Check sheet for the drawn part. Datum: minimum x, y, z corner. Units: mm. A direction names the side the tool comes from. Give positions to 0.01 mm unless a question says otherwise; leave off trailing zeros. Write each loop counter-clockwise with the first axis right and the second up, starting at its lowest first coordinate (ties: lowest second). Pieces come first, ordered by that corner, then holes. Notation, with made-up numbers: (37.25, 72.25) -> (78.25, 72.25) arc R15 cw to (78.25, 79.25) -> close; hole circle Ø9 at (24.25, 89.25). An arc over 180 degrees is marked (long way). Use CSV: the item, a comma, the result in double quotes. Start each with the question number.
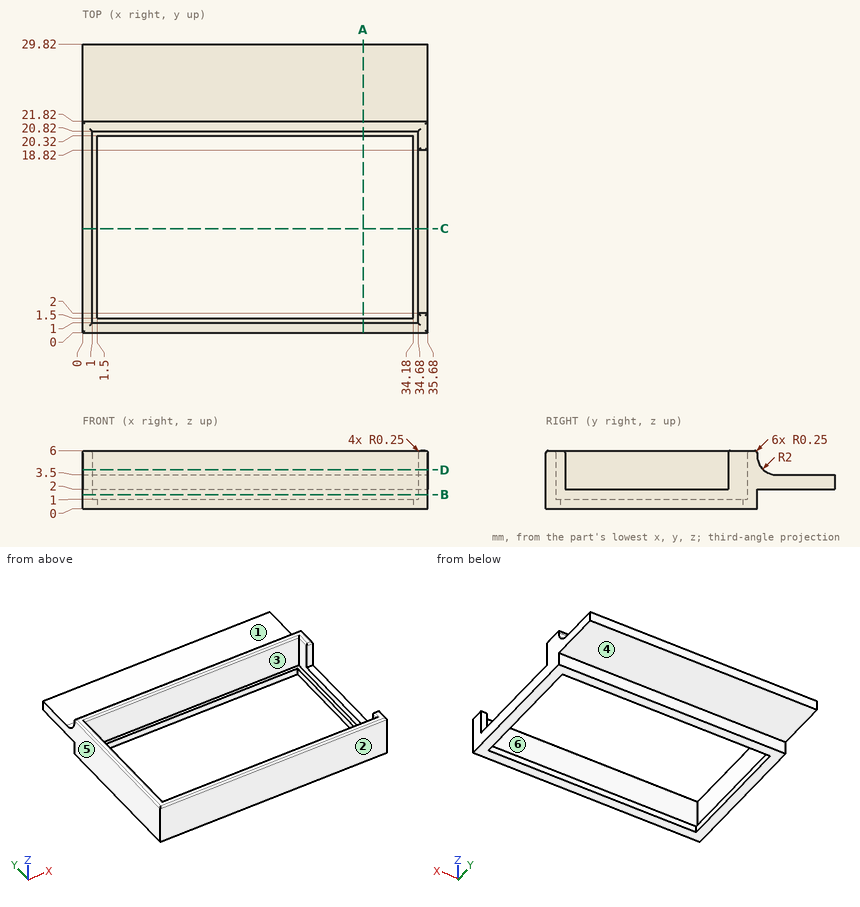
(1) Go/stop test with flat-tipped pins: pin 1 (1.1 mm diameter, centred on x = 35.5, z = 4, fed in from +Y); pin 2 (1.8 mm diameter, centred on x = 23, y = 26.5, fed in from +Z); pin 3 (0.8 mm diameter, centred on x = 23.5, z = 0.5, fed in from +Y); pin 4 (2.5 mm diameter, centred on x = 15.5, y = 25.5, fed in from -Z). Record where each tip stops, or that it passes through.
(2) Section check D-D on z = 4. Record the cut outline in (x, y).
(3) Set-up check for the marked faces 1, 2 and 3: record each of +Z, -Z, +X, -X, +Y, -Y from which the full face is reachable in a straight line by a thin tool's end or side.
(4) Section check A-A on x = 29. Record the cut outline in (y, z).
(5) Draft check along X on the marked faces 4, 5 and 6. Enter one of: released by +X, released by -X, zero draft, split by the parting line, or undercut.
(6) Thickness scan on line 1 (Y direction, x = 27, z = 3.45); line 2 (X direction, y = 9.25, z = 0.85); line 3 (X direction, y = 16.75, z = 1.8). Record the ranges inside material, lowest first. Write a range as from..to.
(7) Section check B-B on z = 1.45. Record the cut outline in (x, y), then the cut area to 3 significant figures.
(8) Section check C-C on y = 10.75. Record the cut outline in (x, z).
Data:
1,pin 1,"stops at y = 29.82"
1,pin 2,"stops at z = 3.5"
1,pin 3,"stops at y = 21.82"
1,pin 4,"stops at z = 2"
2,outline,"(0, 0) -> (35.68, 0) -> (35.68, 2) -> (34.68, 2) -> (34.68, 1) -> (1, 1) -> (1, 20.82) -> (34.68, 20.82) -> (34.68, 18.82) -> (35.68, 18.82) -> (35.68, 22.5) -> (0, 22.5) -> close"
3,face 1,"+Z, +X, -X, +Y"
3,face 2,"+Z, -Z, +X, -X, -Y"
3,face 3,"+Z"
4,outline,"(0, 0) -> (1.5, 0) -> (1.5, 1) -> (1, 1) -> (1, 5.75) arc R0.25 ccw to (0.75, 6) -> (0.25, 6) arc R0.25 ccw to (0, 5.75) -> close; (20.32, 0) -> (21.82, 0) -> (21.82, 2) -> (29.82, 2) -> (29.82, 3.5) -> (23.82, 3.5) arc R2 cw to (21.82, 5.5) -> (21.82, 5.75) arc R0.25 ccw to (21.57, 6) -> (21.07, 6) arc R0.25 ccw to (20.82, 5.75) -> (20.82, 1) -> (20.32, 1) -> close"
5,face 4,"zero draft"
5,face 5,"released by -X"
5,face 6,"undercut"
6,line 1,"y = 0..1, 20.82..29.82"
6,line 2,"x = 0..1.5, 34.18..35.68"
6,line 3,"x = 0..1, 34.68..35.68"
7,outline,"(0, 0) -> (35.68, 0) -> (35.68, 21.82) -> (0, 21.82) -> close; hole (1, 1) -> (34.68, 1) -> (34.68, 20.82) -> (1, 20.82) -> close"
7,area,"111 mm2"
8,outline,"(0, 0) -> (1.5, 0) -> (1.5, 1) -> (1, 1) -> (1, 5.75) arc R0.25 ccw to (0.75, 6) -> (0.25, 6) arc R0.25 ccw to (0, 5.75) -> close; (34.18, 0) -> (35.68, 0) -> (35.68, 2) -> (34.68, 2) -> (34.68, 1) -> (34.18, 1) -> close"
